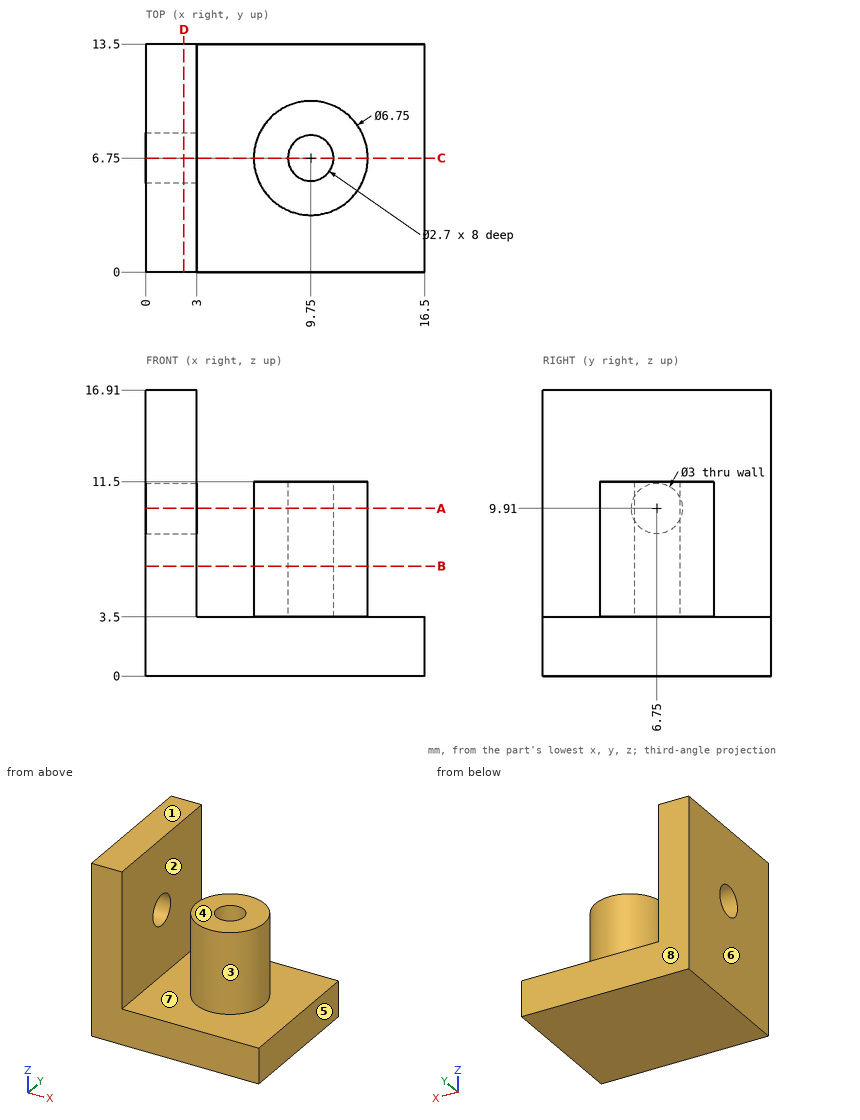
Input: dimensioned drawing with shaded views. Units: mm. Origin: part minimum x, y, z. A direction names the side the tool comes from. Round coordinates to 2 decimals unless told otherwise and drop trailing zeros. Loops run counter-clockwise (first coordinate to the right, second up) from the corner with the lowest first, then second, coordinate; pieces in that order, holes last. Notation, with made-up numbers: (-17.75, 85.25) -> (29.25, 85.25) arc R23 ccw to (29.25, 96.25) -> close; hole circle Ø2 at (17.25, 14.5). An arc over 180 degrees is marked (long way). Use one line per item in the form item = value. Start each with the question number.
1) Section C-C on y = 6.75. Output: boundary loops of the cut face in (x, z) (3 decimals).
2) Line query: L1, parallel to Y at x = 9.75, z = 8 (3 decimals); L2, parallel to Z at x = 2.45, y = 6.75; L3, parallel to X at y = 3.75, z = 15.25. Output: solid intervals per line, ascending.
3) Draft query along X for the marked faces 6, 7 and 8. Return one class per face: released by +X, released by -X, zero draft, split by the parting line, or undercut.
4) First-contact query: P1, Ø8, axis at y = 1.5, z = 9, coming from the +X side (3 decimals); P2, Ø5, axis at x = 14.5, z = 15, coming from the +Y side; P3, Ø2, axis at x = 8.5, z = 11, coming from the -Y side; P4, Ø5.5, axis at x = 10, y = 5.5, coming from the +Z side. Flat tips, straight axial feed; report the tip coordinate or a pass-through.
5) Section B-B on z = 6.5. Output: boundary loops of the cut face in (x, y) (3 decimals), then the cut area to 3 significant figures.
6) Section D-D on x = 2.25. Output: boundary loops of the cut face in (y, z), then the cut area to 3 significant figures.
7) Access query for the marked faces 1, 2, 3, 4 and 5. Directions: +Z, -Z, +X, -X, +Y, -Y. A direction counts if a zero-diameter tool reaches every point of the face in a straight line with its end or side. Return the directions, or none.
8) Section A-A on z = 9.91. Output: boundary loops of the cut face in (x, y) (3 decimals).
Response:
q1.outline = (0, 0) -> (16.5, 0) -> (16.5, 3.5) -> (13.125, 3.5) -> (13.125, 11.5) -> (11.1, 11.5) -> (11.1, 3.5) -> (8.4, 3.5) -> (8.4, 11.5) -> (6.375, 11.5) -> (6.375, 3.5) -> (3, 3.5) -> (3, 8.41) -> (0, 8.41) -> close; (0, 11.41) -> (3, 11.41) -> (3, 16.91) -> (0, 16.91) -> close
q2.L1 = 3.375 to 5.4, 8.1 to 10.125
q2.L2 = 0 to 8.41, 11.41 to 16.91
q2.L3 = 0 to 3
q3.face_6 = released by -X
q3.face_7 = undercut
q3.face_8 = zero draft
q4.P1 = 12.885
q4.P2 = through
q4.P3 = 3.38
q4.P4 = 11.5
q5.outline = (0, 0) -> (3, 0) -> (3, 13.5) -> (0, 13.5) -> close; circle Ø6.75 at (9.75, 6.75); hole circle Ø2.7 at (9.75, 6.75)
q5.area = 70.6 mm^2
q6.outline = (0, 0) -> (13.5, 0) -> (13.5, 16.91) -> (0, 16.91) -> close; hole circle Ø3 at (6.75, 9.91)
q6.area = 221 mm^2
q7.face_1 = +Z, +X, -X, +Y, -Y
q7.face_2 = +Z, +Y, -Y
q7.face_3 = +Z
q7.face_4 = +Z, +X, +Y, -Y
q7.face_5 = +Z, -Z, +X, +Y, -Y
q8.outline = (0, 0) -> (3, 0) -> (3, 5.25) -> (0, 5.25) -> close; (0, 8.25) -> (3, 8.25) -> (3, 13.5) -> (0, 13.5) -> close; circle Ø6.75 at (9.75, 6.75); hole circle Ø2.7 at (9.75, 6.75)
